Could you check a few things on this model? Use its own coordinates, in mm. A direction names the side the tool comes from. Coordinates: 2 decimals unless noted, no trailing zeros. Loops run counter-clockwise (first coordinate to the right, second up) from the corner with the lowest first, then second, coordinate; pieces in that order, holes last. Notation, with made-up numbers: (5.25, 55.25) -> (56.25, 55.25) arc R28 cw to (56.25, 83.25) -> close; hole circle Ø5 at (-19.75, 15). An arc over 180 degrees is marked (long way). One line per question, with ' | ' between items.
```python
from build123d import *

# Parameters (mm, degrees)
F0_W     = 70
F0_H     = 20
F1_DEPTH = 15
F3_T     = -1
F4_D     = 5
F2_W     = 35
F2_H     = 5
F5_DEPTH = 25
F6_R     = 2.49999


# Not quite as in the source:
# - a fillet or chamfer is up to 0.001 mm smaller than in the source, because OpenCascade refuses the exact size


with BuildPart() as f1:
    # F0 (on Top) → F1 (new body)
    with BuildSketch(Plane.XY):
        with Locations((0, 1.5861968277)):
            Rectangle(F0_W, F0_H)
    extrude(amount=F1_DEPTH)

    # F3
    f3_openings = [f1.faces().sort_by_distance(p)[0] for p in [
        (0, 1.586197, 15),
    ]]
    offset(amount=F3_T, openings=f3_openings)

    # F4 (through all)
    with Locations(Plane.XZ.offset(8.4138031723)):
        with Locations((-28.8131628186, 7.5)):
            Hole(F4_D / 2)

    # F2 (on face) → F5 (cut)
    with BuildSketch(Plane.XZ.offset(8.4138031723)):
        with Locations((4.5323091745, 7.627816461)):
            Rectangle(F2_W, F2_H)
    extrude(amount=-F5_DEPTH, mode=Mode.SUBTRACT)

    # F6 (radius 2.5 in the source; OpenCascade refuses exactly that, so slightly less here)
    f6_edges = [f1.edges().sort_by_distance(p)[0] for p in [
        (-12.967691, -7.913803, 10.127816),
        (-12.967691, -7.913803, 5.127816),
        (22.032309, -7.913803, 5.127816),
        (22.032309, -7.913803, 10.127816),
    ]]
    fillet(f6_edges, radius=F6_R)


solid = f1.part
```
Q1. Imagine slicing it at C-C on y = 3. Write out the boundary of the cut face in (x, z), plus the area to 3 significant figures.
Values follow:
outline: (-35, 0) -> (35, 0) -> (35, 15) -> (34, 15) -> (34, 1) -> (-34, 1) -> (-34, 15) -> (-35, 15) -> close | area: 98.0 mm2
Q2. Imagine slicing it at B-B on x = -20.5. Write out the boundary of the cut face in (y, z).
Values follow:
outline: (-8.41, 0) -> (11.59, 0) -> (11.59, 15) -> (10.59, 15) -> (10.59, 1) -> (-7.41, 1) -> (-7.41, 15) -> (-8.41, 15) -> close
Q3. We'd pull the mould along Y, two halves only. Please class faces 1 (the face through (0, -8.414, 4)), 2 (the face through (0, 2, 0)), 3 (the face through (-34, 1, 8)): released by +Y, released by -Y, zero draft, split by the parting line, or undercut.
Values follow:
face 1: released by -Y | face 2: zero draft | face 3: undercut
Q4. For faces 4 (the face through (35, 1, 7)), 5 (the face through (34, 1, 8)), 6 (the face through (-12.255, -7.907, 5.88)), which set-ups out of +Z, -Z, +X, -X, +Y, -Y let a thin tool reach every point of the face, with its end or its side?
Values follow:
face 4: +Z, -Z, +X, +Y, -Y | face 5: +Z | face 6: +Y, -Y
Q5. Imagine slicing it at D-D on x = 8. Write out the boundary of the cut face in (y, z).
Values follow:
outline: (-8.41, 0) -> (11.59, 0) -> (11.59, 5.13) -> (10.59, 5.13) -> (10.59, 1) -> (-7.41, 1) -> (-7.41, 5.13) -> (-8.41, 5.13) -> close; (-8.41, 10.13) -> (-7.41, 10.13) -> (-7.41, 15) -> (-8.41, 15) -> close; (10.59, 10.13) -> (11.59, 10.13) -> (11.59, 15) -> (10.59, 15) -> close
Q6. Imagine slicing it at A-A on z = 3.75. Write out the boundary of the cut face in (x, y).
Values follow:
outline: (-35, -8.41) -> (35, -8.41) -> (35, 11.59) -> (-35, 11.59) -> close; hole (-34, -7.41) -> (34, -7.41) -> (34, 10.59) -> (-34, 10.59) -> close
Q7. For pin 1 (8 mm diameter, centred on x = 5.5, y = 5.5, fed in from +Z), with a flat end and sliding along its axis, tell me the tip position at first contact or that it passes through.
Values follow:
pin 1: stops at z = 1
Q8. Please list where these lines run through material, in increasing order: L1, parallel to X at y = -2.25, z = 8; L2, parallel to Y at x = 2, z = 12.5; L3, parallel to Z at x = 17, y = -2. Write a range as [from, to].
Values follow:
L1: x = [-35, -34], [34, 35] | L2: y = [-8.41, -7.41], [10.59, 11.59] | L3: z = [0, 1]
